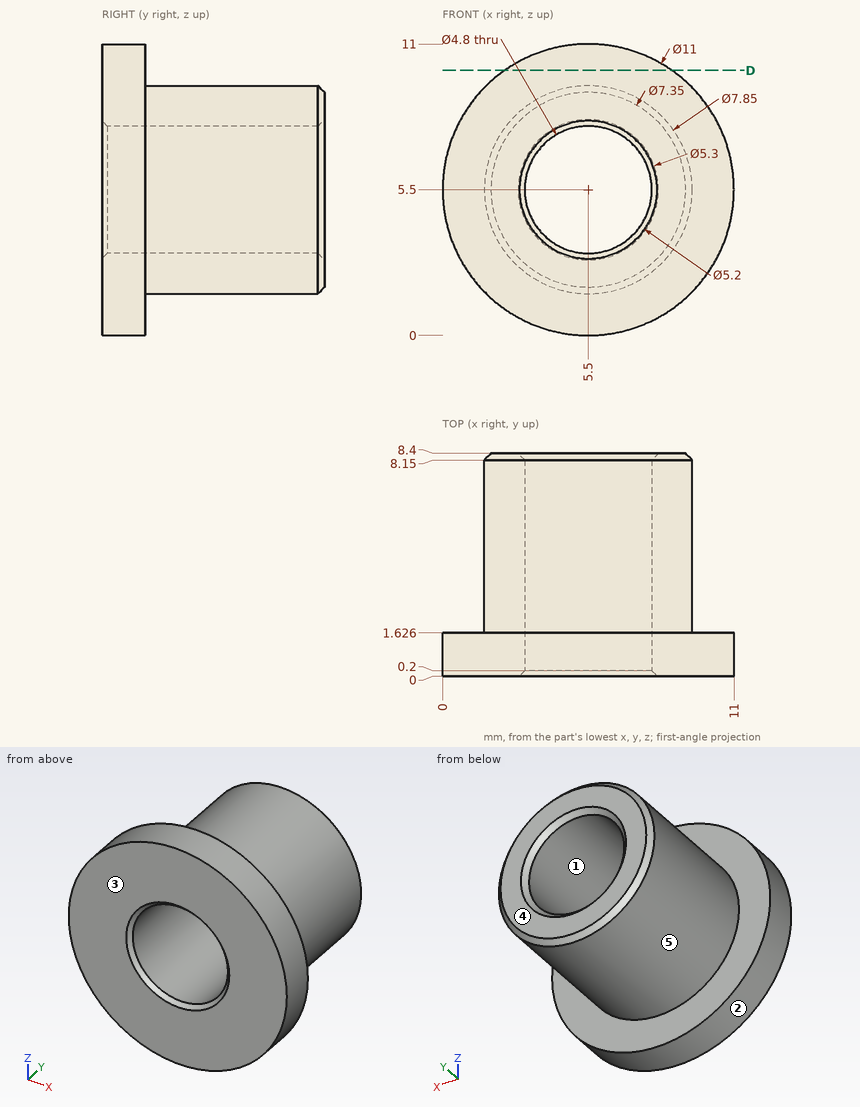
Source: three-view drawing plus pictorial views. Frame: mm from the lowest corner of the part. A direction names the side the tool comes from. Give positions to 0.01 mm unless a question says otherwise; leave off trailing zeros. Order: outer loops, then holes, each group sorted by start corner. A loop starts at its lowest first (then second) coordinate and runs counter-clockwise, first axis right, second up. Notation, with made-up numbers: M 8,-7 L 26,-7 A17 ccw 26,12 Z; hole C 76,-31 d11. An arc over 180 degrees is marked long. Return JSON: item names as keys, results as strings.
Item 1: Pull-direction query (X, two-part tool) for the marked faces 1, 2 and 3; classes: +X half, -X half, draft (parallel to the pull), parting line (faces both ways), or undercut.
Solutions:
{"face 1": "undercut", "face 2": "parting line", "face 3": "draft"}
Item 2: Ray query, probe 1 along Z at (x, y) = (5.5, 2) (1 decimal); probe 2 along Y at (x, z) = (9, 3) (1 decimal); probe 3 along Z at (x, y) = (4.75, 2.25). Return the intervals inside material, ascending.
Solutions:
{"probe 1": "1.6 to 3.1, 7.9 to 9.4", "probe 2": "0 to 1.6", "probe 3": "1.65 to 3.22, 7.78 to 9.35"}
Item 3: Cut plane D-D (z = 10). Return loops of the section in (x, y) (1 decimal).
Solutions:
{"outline": "M 2.3,0 L 8.7,0 L 8.7,1.6 L 2.3,1.6 Z"}
Item 4: Access query for the marked faces 4 and 5. Directions: +Z, -Z, +X, -X, +Y, -Y. A direction counts if a zero-diameter tool reaches every point of the face in a straight line with its end or side. Return the directions, or none.
Solutions:
{"face 4": "+Z, -Z, +X, -X, +Y", "face 5": "+Y"}
Item 5: First-contact query: P1, Ø1.5, axis at x = 6, z = 1, coming from the +Y side; P2, Ø4, axis at y = 3.5, z = 7.5, coming from the -X side; P3, Ø5, axis at y = 3, z = 8.5, coming from the -X side. Flat tips, straight axial feed; report the tip coordinate or a pass-through.
Solutions:
{"P1": "y = 8.3", "P2": "x = 0.16", "P3": "x = 0.08"}
